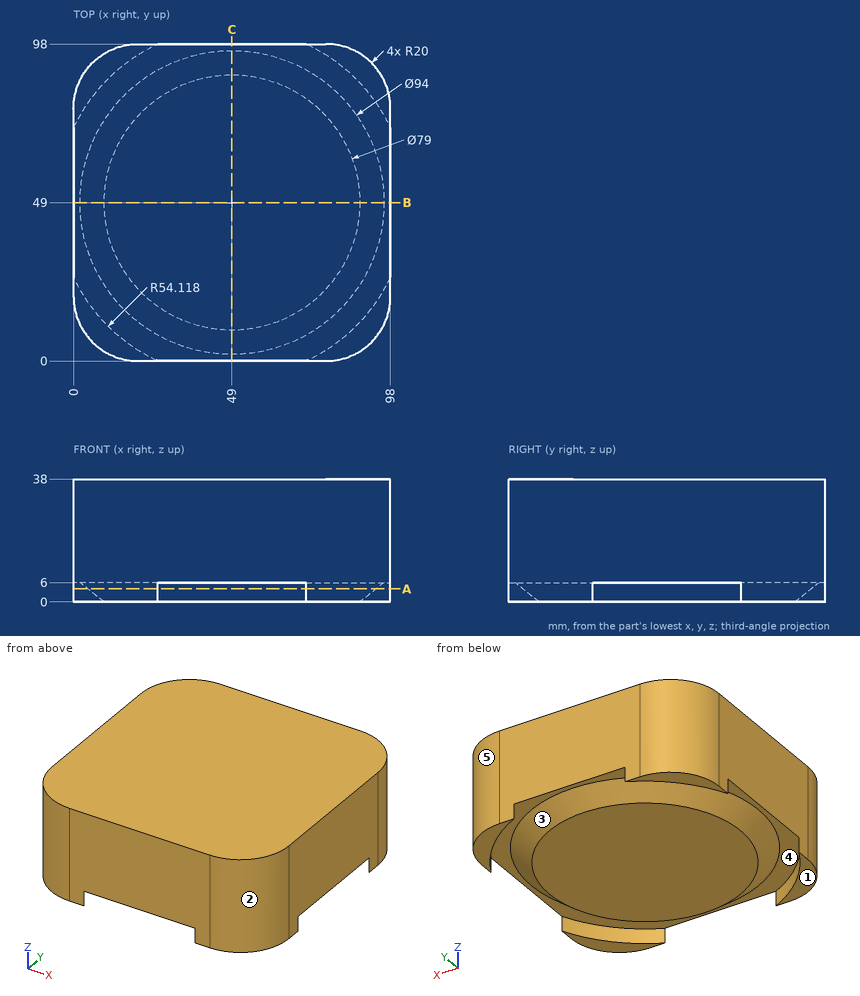
Here's the drawing with two shaded views (mm, measured from the low corner). I have some questions. A direction names the side the tool comes from. Give positions to 0.01 mm unless a question says otherwise; leave off trailing zeros. Order: outer loops, then holes, each group sorted by start corner. A loop starts at its lowest first (then second) coordinate and runs counter-clockwise, first axis right, second up. Notation, with made-up numbers: (-7.5, 86) -> (9.5, 86) arc R20 cw to (9.5, 103) -> close; hole circle Ø3 at (-24.5, 63). An arc over 180 degrees is marked (long way). One line per item, written item: value. Start each with the question number.
1. Imagine slicing it at B-B, the plane y = 49. List the corners of the cut face in (x, z) for me, plus the area to 4 significant figures.
2. Imagine slicing it at A-A, the plane z = 4. List the corners of the cut face in (x, y) for me (1 decimal).
3. We'd pull the mould along Y, two halves only. Please class the marked faces 1, 2 and 3: released by +Y, released by -Y, zero draft, split by the parting line, or undercut.
4. For the marked faces 4 and 5, which set-ups out of +Z, -Z, +X, -X, +Y, -Y let a thin tool reach every point of the face, with its end or its side?
5. I need wall thicknesses on probe 1 along Z at (x, y) = (5, 21.5); probe 2 along X at (y, z) = (19.5, 28); probe 3 along X at (y, z) = (85.5, 19). Which ranges of each line are inside material? Lowest first, please. Write a range as from..to.
Values follow:
1. outline: (0, 6) -> (2, 6) -> (9.5, 0) -> (88.5, 0) -> (96, 6) -> (98, 6) -> (98, 38) -> (0, 38) -> close
1. area: 3,655 mm2
2. outline: (0, 20) arc R20 ccw to (20, 0) -> (26, 0) arc R54.1 cw to (0, 26) -> close; (0, 72) arc R54.1 cw to (26, 98) -> (20, 98) arc R20 ccw to (0, 78) -> close; circle Ø89 at (49, 49); (72, 0) -> (78, 0) arc R20 ccw to (98, 20) -> (98, 26) arc R54.1 cw to start; (72, 98) arc R54.1 cw to (98, 72) -> (98, 78) arc R20 ccw to (78, 98) -> close
3. face 1: zero draft
3. face 2: released by -Y
3. face 3: undercut
4. face 4: -Z
4. face 5: +Z, -Z, +X, +Y
5. probe 1: z = 6..38
5. probe 2: x = 0.01..97.99
5. probe 3: x = 1.46..96.54
